```python
from build123d import *

# Parameters (mm, degrees)
SKETCH1_R           = 2.4511
SKETCH1_R_2         = 3.429
BOSS_EXTRUDE1_DEPTH = 6.35
FILLET1_R           = 3.175


with BuildPart() as part:
    # Sketch1 → Boss-Extrude1 (new body)
    with BuildSketch(Plane(origin=(0, 0, 0), x_dir=(0, 0, -1), z_dir=(1, 0, 0))):
        Polygon((0, 0), (-38.1, 0), (-57.15, 50.8), (-146.05, 50.8), (-146.05, 114.3), (0, 114.3), align=None)
        with Locations((-19.05, 101.6)):
            Circle(SKETCH1_R, mode=Mode.SUBTRACT)
        with Locations((-19.05, 69.85)):
            Circle(SKETCH1_R, mode=Mode.SUBTRACT)
        with Locations((-19.05, 38.1)):
            Circle(SKETCH1_R, mode=Mode.SUBTRACT)
        with Locations((-19.05, 6.35)):
            Circle(SKETCH1_R, mode=Mode.SUBTRACT)
        with Locations((-53.975, 101.6)):
            Circle(SKETCH1_R_2, mode=Mode.SUBTRACT)
        with Locations((-89.027, 101.6)):
            Circle(SKETCH1_R_2, mode=Mode.SUBTRACT)
        with Locations((-89.027, 63.5)):
            Circle(SKETCH1_R_2, mode=Mode.SUBTRACT)
        with Locations((-53.975, 63.5)):
            Circle(SKETCH1_R_2, mode=Mode.SUBTRACT)
    extrude(amount=BOSS_EXTRUDE1_DEPTH)

    # Fillet1
    fillet1_edges = [part.edges().sort_by_distance(p)[0] for p in [
        (3.175, 0, 0),
        (3.175, 0, 38.1),
        (3.175, 50.8, 57.15),
        (3.175, 50.8, 146.05),
        (3.175, 114.3, 146.05),
        (3.175, 114.3, 0),
    ]]
    fillet(fillet1_edges, radius=FILLET1_R)


solid = part.part
```
CAD build for the part. Positions are in the model's coordinates, mm. Give positions to 0.01 mm unless a question says otherwise; leave off trailing zeros. Order: outer loops, then holes, each group sorted by start corner. A loop starts at its lowest first (then second) coordinate and runs counter-clockwise, first axis right, second up. Notation, with made-up numbers: M -17.5,-25 L 37.5,-25 A36 ccw 37.5,9 Z; hole C 30.5,67 d7. An arc over 180 degrees is marked long. Put each result on its own line as item: value. Start each with the question number.
(1) Drill centre lines: line 1 along Y through (x, z) = (2.25, 19.05); line 2 along Z through (x, y) = (4.5, 99.5); line 3 along Y through (x, z) = (1, 111). Where is each one in solid material? Low to high.
(2) Saw through at B-B, the plane z = 19.05. Write the cut outline in (x, y), then the cut area to 3 significant figures.
(3) Flat gauge pins, fed straight in: pin 1 Ø6 at (y, z) = (63.5, 53.975) entering from +X; pin 2 Ø2 at (x, z) = (4.5, 97.5) entering from -Y. Where does each tip first touch, or does it go through?
(4) Saw through at C-C, the plane x = 4.5. Give the number of separate pieces and of enclosed holes in the cut face, then the cut area to 3 significant figures.
(5) Saw through at A-A, the plane y = 69.85. Write the cut outline in (x, z).
(6) Saw through at D-D, the plane y = 101.6. Write the cut outline in (x, z), then the cut area to 3 significant figures.
(7) Mould opens along Y. For faces 1 (the flat face through (3.13, 25.07, 47.5)), 2 (the cylindrical face through (3.131, 60.153, 54.718)), 3 (the flat face through (0, 71, 56)) say: +Y half, -Y half, draft (parallel to the pull), parting line (faces both ways), or undercut.
Check result:
1. line 1: y = 0 to 3.9, 8.8 to 35.65, 40.55 to 67.4, 72.3 to 99.15, 104.05 to 114.3
1. line 2: z = 0 to 17.79, 20.31 to 51.26, 56.69 to 86.32, 91.74 to 146.05
1. line 3: y = 50.8 to 114.3
2. outline: M 0,0 L 6.35,0 L 6.35,3.9 L 0,3.9 Z; M 0,8.8 L 6.35,8.8 L 6.35,35.65 L 0,35.65 Z; M 0,40.55 L 6.35,40.55 L 6.35,67.4 L 0,67.4 Z; M 0,72.3 L 6.35,72.3 L 6.35,99.15 L 0,99.15 Z; M 0,104.05 L 6.35,104.05 L 6.35,114.3 L 0,114.3 Z
2. area: 601 mm2
3. pin 1: passes through
3. pin 2: stops at y = 50.8
4. separate pieces: 1
4. enclosed holes: 8
4. area: 11,500 mm2
5. outline: M 0,0 L 6.35,0 L 6.35,16.6 L 0,16.6 Z; M 0,21.5 L 6.35,21.5 L 6.35,146.05 L 0,146.05 Z
6. outline: M 0,0 L 6.35,0 L 6.35,16.6 L 0,16.6 Z; M 0,21.5 L 6.35,21.5 L 6.35,50.55 L 0,50.55 Z; M 0,57.4 L 6.35,57.4 L 6.35,85.6 L 0,85.6 Z; M 0,92.46 L 6.35,92.46 L 6.35,146.05 L 0,146.05 Z
6. area: 809 mm2
7. face 1: -Y half
7. face 2: undercut
7. face 3: draft
